Design review of the part built by this model. Coordinates are the model's own, in mm. Face numbers are marked on the shaded views. Give positions to 0.01 mm unless a question says otherwise; leave off trailing zeros. Order: outer loops, then holes, each group sorted by start corner. A loop starts at its lowest first (then second) coordinate and runs counter-clockwise, first axis right, second up.
```python
from build123d import *

# Parameters (mm, degrees)
BOSS_EXTRUDE1_DEPTH         = 90
BOSS_EXTRUDE2_DEPTH         = 90
CUT_EXTRUDE1_REACH          = 102.574
SKETCH5_W                   = 62.668099026
SKETCH5_H                   = 5.35
TAP_DRILL_FOR_M5X0_8_TAP1_D = 4.2


with BuildPart() as part:
    # Sketch1 → Boss-Extrude1 (new body)
    with BuildSketch(Plane.XY):
        with BuildLine():
            Line((-31.734248061, 1), (-17.721808598, 1))
            ThreePointArc((-17.721808598, 1), (0, 17.75), (17.721808598, 1))
            Line((17.721808598, 1), (31.734248061, 1))
            ThreePointArc((31.734248061, 1), (0, 31.75), (-31.734248061, 1))
        make_face()
    extrude(amount=BOSS_EXTRUDE1_DEPTH)

    # Sketch4 → Boss-Extrude2 (add)
    with BuildSketch(Plane(origin=(0, 0, 0), x_dir=(-1, 0, 0), z_dir=(0, 0, -1))):
        with BuildLine():
            Line((-30.765263387, 31.75), (-31.734248061, 1))
            ThreePointArc((-31.734248061, 1), (-22.094258304, 22.801452805), (0, 31.75))
            Line((0, 31.75), (-30.765263387, 31.75))
        make_face()
        with BuildLine():
            Line((31.734248061, 31.75), (0, 31.75))
            ThreePointArc((0, 31.75), (22.094258304, 22.801452805), (31.734248061, 1))
            Line((31.734248061, 1), (31.734248061, 31.75))
        make_face()
    extrude(amount=-BOSS_EXTRUDE2_DEPTH)

    # Sketch5 → Cut-Extrude1 (cut, up to next)
    with BuildSketch(Plane.XY.offset(90), mode=Mode.PRIVATE) as cut_extrude1_sk1:
        with Locations((-0.400198548, 29.075)):
            Rectangle(SKETCH5_W, SKETCH5_H)
    cut_extrude1_tool1 = extrude(cut_extrude1_sk1.sketch, amount=-CUT_EXTRUDE1_REACH, mode=Mode.PRIVATE) & part.part
    add(cut_extrude1_tool1.solids().sort_by_distance((-0.400199, 29.075, 90))[0], mode=Mode.SUBTRACT)

    # Tap Drill for M5x0.8 Tap1 (through all)
    with Locations(Plane(origin=(-24.72802833, 1, 80), x_dir=(0, 0, -1), z_dir=(0, -1, 0))):
        with Locations((0, 0), (70, 0), (0, 49.45605666), (70, 49.45605666)):
            Hole(TAP_DRILL_FOR_M5X0_8_TAP1_D / 2)


solid = part.part
```
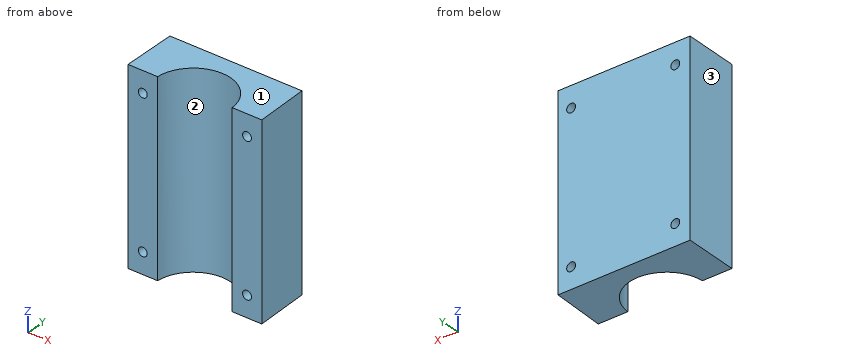
1. For pin 1 (1.5 mm diameter, centred on y = 4.5, z = 25.5, fed in from +X), flat-tipped, find the tip position at first contact; note if it passes through.
Recorded:
pin 1: stops at x = 31.65
2. Take a section at B-B (z = 80). State the section outline as (x, y) points.
Recorded:
outline: (-31.73, 1) - (-26.83, 1) - (-26.83, 26.4) - (-31.73, 26.4) - close; (-22.63, 1) - (-17.72, 1) arc R17.75 cw to (17.72, 1) - (22.63, 1) - (22.63, 26.4) - (-22.63, 26.4) - close; (26.83, 1) - (31.73, 1) - (30.93, 26.4) - (26.83, 26.4) - close
3. Draft analysis for pull direction X (two halves, no side actions). For the marked faces 1, 2 and 3, state which applies: pulls with the +X half, pulls with the -X half, needs draft (parallel to the pull), parting line crosses it, or undercut.
Recorded:
face 1: needs draft
face 2: undercut
face 3: pulls with the -X half
4. Take a section at D-D (x = 0). State the section outline as (y, z) points, then the cut area to 4 significant figures.
Recorded:
outline: (17.75, 0) - (26.4, 0) - (26.4, 90) - (17.75, 90) - close
area: 778.5 mm2
5. Take a section at C-C (y = 22.5). State the section outline as (x, z) points.
Recorded:
outline: (-31.73, 0) - (31.06, 0) - (31.06, 90) - (-31.73, 90) - close; hole circle Ø4.2 at (-24.73, 10); hole circle Ø4.2 at (-24.73, 80); hole circle Ø4.2 at (24.73, 10); hole circle Ø4.2 at (24.73, 80)
6. For line 1 along X through (y, z) = (7.5, 10); line 2 along X through (y, z) = (7.75, 80); line 3 along X through (y, z) = (4.25, 48), list the stretches that pass through material, from the lowest coordinate up.
Recorded:
line 1: x = -31.73 to -26.83, -22.63 to -16.09, 16.09 to 22.63, 26.83 to 31.53
line 2: x = -31.73 to -26.83, -22.63 to -15.97, 15.97 to 22.63, 26.83 to 31.52
line 3: x = -31.73 to -17.23, 17.23 to 31.63
7. Take a section at A-A (y = 14). State the section outline as (x, z) points, then the cut area to 3 significant figures.
Recorded:
outline: (-31.73, 0) - (-10.91, 0) - (-10.91, 90) - (-31.73, 90) - close; (10.91, 0) - (31.32, 0) - (31.32, 90) - (10.91, 90) - close; hole circle Ø4.2 at (-24.73, 10); hole circle Ø4.2 at (-24.73, 80); hole circle Ø4.2 at (24.73, 10); hole circle Ø4.2 at (24.73, 80)
area: 3,660 mm2
